Source: CAD feature listing. Evaluate the final solid. Frame: model axes, mm. A direction names the side the tool comes from. Coordinates: 2 decimals unless noted, no trailing zeros. Loops run counter-clockwise (first coordinate to the right, second up) from the corner with the lowest first, then second, coordinate; pieces in that order, holes last. Notation, with made-up numbers: M 2.25,31.5 L 6.25,31.5 A30 cw 6.25,66.5 Z; hole C -33,57 d9. An arc over 180 degrees is marked long. One line per question, with ' | ' between items. Start each with the question number.
1. Section query C-C, the plane z = 2.75. Output: boundary loops of the cut face in (x, y).
2. Section query B-B, the plane y = 30. Output: boundary loops of the cut face in (x, z), and give its area (3 significant figures).
3. Pin query (flat end, axial travel): P1, Ø5, axis at x = 31, y = -31, coming from the +Z side; P2, Ø1.5, axis at x = 9.5, z = 5, coming from the -Y side; P3, Ø5, axis at x = 29.5, y = 33, coming from the +Z side. Return the tip coordinate at first contact, or that it passes through.
4. Access query for faces 1 (the cylindrical face through (-27, 30.1, 0.5)), 2 (the cylindrical face through (-30.1, 23.5, 3.5)). Directions: +Z, -Z, +X, -X, +Y, -Y. A direction counts if a zero-diameter tool reaches every point of the face in a straight line with its end or side. Return the directions, or none.
5. Section query D-D, the plane y = -12.8. Output: boundary loops of the cut face in (x, z), and give its area (3 significant figures).
6. Ray query, probe 1 along Y at (x, z) = (-30, 0.65); probe 2 along X at (y, z) = (-31, 1.75); probe 3 along Y at (x, z) = (0, 2.75). Return the intervals inside material, ascending.
7. Mould query, pull axis Y, two halves, no side actions, for faces 3 (the cylindrical face through (-29.9, -23.5, 3.5)), 4 (the flat face through (41.5, -0.6, 5)), 5 (the flat face through (-1, 42.5, 2)). Classes: pulls with the +Y half, pulls with the -Y half, needs draft (parallel to the pull), parting line crosses it, or undercut.
8. Section query A-A, the plane x = -30. Output: boundary loops of the cut face in (y, z), and give its area (3 significant figures).
```python
from build123d import *

# Parameters (mm, degrees)
F0_W     = 85
F0_H     = 85
F1_DEPTH = 6
F2_R     = 5.5
F3_DEPTH = 6.001
F5_D     = 6
F6_SIZE  = 2
F8_DEPTH = 5


with BuildPart() as f1:
    # F0 (on Top) → F1 (new body)
    with BuildSketch(Plane.XY):
        Rectangle(F0_W, F0_H)
    extrude(amount=F1_DEPTH)

    # F2 (on face) → F3 (cut, through all)
    with BuildSketch(Plane.XY.offset(6)):
        with Locations((0, 12.8)):
            Circle(F2_R)
        with Locations((0, -12.8)):
            Circle(F2_R)
    extrude(amount=-F3_DEPTH, mode=Mode.SUBTRACT)

    # F5 (through all)
    with Locations(Plane.XY.offset(6)):
        with Locations((-30, -30), (-30, 30), (30, 30), (30, -30)):
            Hole(F5_D / 2)

    # F6
    f6_edges = [f1.edges().sort_by_distance(p)[0] for p in [
        (-42.5, 0, 6),
        (0, -42.5, 6),
        (42.5, 0, 6),
        (0, 42.5, 6),
    ]]
    chamfer(f6_edges, length=F6_SIZE)

    # F7 (on face) → F8 (cut)
    with BuildSketch(Plane.XY.offset(6)):
        with BuildLine():
            ThreePointArc((33.25, 33.25), (30, 36.5), (26.75, 33.25))
            Line((26.75, 33.25), (26.75, 26.75))
            ThreePointArc((26.75, 26.75), (30, 23.5), (33.25, 26.75))
            Line((33.25, 26.75), (33.25, 33.25))
        make_face()
        with BuildLine():
            Line((-26.75, 26.75), (-26.75, 33.25))
            ThreePointArc((-26.75, 33.25), (-30, 36.5), (-33.25, 33.25))
            Line((-33.25, 33.25), (-33.25, 26.75))
            ThreePointArc((-33.25, 26.75), (-30, 23.5), (-26.75, 26.75))
        make_face()
        with BuildLine():
            Line((26.75, -26.75), (26.75, -33.25))
            ThreePointArc((26.75, -33.25), (30, -36.5), (33.25, -33.25))
            Line((33.25, -33.25), (33.25, -26.75))
            ThreePointArc((33.25, -26.75), (30, -23.5), (26.75, -26.75))
        make_face()
        with BuildLine():
            ThreePointArc((-33.25, -33.25), (-30, -36.5), (-26.75, -33.25))
            Line((-26.75, -33.25), (-26.75, -26.75))
            ThreePointArc((-26.75, -26.75), (-30, -23.5), (-33.25, -26.75))
            Line((-33.25, -26.75), (-33.25, -33.25))
        make_face()
    extrude(amount=-F8_DEPTH, mode=Mode.SUBTRACT)


solid = f1.part
```
Taken from the geometry:
1) outline: M -42.5,-42.5 L 42.5,-42.5 L 42.5,42.5 L -42.5,42.5 Z; hole M -33.25,-33.25 A3.25 ccw -26.75,-33.25 L -26.75,-26.75 A3.25 ccw -33.25,-26.75 Z; hole M -33.25,26.75 A3.25 ccw -26.75,26.75 L -26.75,33.25 A3.25 ccw -33.25,33.25 Z; hole C 0,-12.8 d11; hole C 0,12.8 d11; hole M 26.75,-33.25 A3.25 ccw 33.25,-33.25 L 33.25,-26.75 A3.25 ccw 26.75,-26.75 Z; hole M 26.75,26.75 A3.25 ccw 33.25,26.75 L 33.25,33.25 A3.25 ccw 26.75,33.25 Z
2) outline: M -42.5,0 L -33,0 L -33,1 L -33.25,1 L -33.25,6 L -40.5,6 L -42.5,4 Z; M -27,0 L 27,0 L 27,1 L 26.75,1 L 26.75,6 L -26.75,6 L -26.75,1 L -27,1 Z; M 33,0 L 42.5,0 L 42.5,4 L 40.5,6 L 33.25,6 L 33.25,1 L 33,1 Z | area: 429 mm^2
3) P1: z = 6 | P2: y = -42.25 | P3: z = 1
4) face 1: +Z, -Z | face 2: +Z
5) outline: M -42.5,0 L -5.5,0 L -5.5,6 L -40.5,6 L -42.5,4 Z; M 5.5,0 L 42.5,0 L 42.5,4 L 40.5,6 L 5.5,6 Z | area: 440 mm^2
6) probe 1: -42.5 to -33, -27 to 27, 33 to 42.5 | probe 2: -42.5 to -33.25, -26.75 to 26.75, 33.25 to 42.5 | probe 3: -42.5 to -18.3, -7.3 to 7.3, 18.3 to 42.5
7) face 3: undercut | face 4: needs draft | face 5: pulls with the +Y half
8) outline: M -42.5,0 L -33,0 L -33,1 L -36.5,1 L -36.5,6 L -40.5,6 L -42.5,4 Z; M -27,0 L 27,0 L 27,1 L 23.5,1 L 23.5,6 L -23.5,6 L -23.5,1 L -27,1 Z; M 33,0 L 42.5,0 L 42.5,4 L 40.5,6 L 36.5,6 L 36.5,1 L 33,1 Z | area: 364 mm^2
